The listing builds one solid part. Answer for the finished solid, in the listing's coordinates (mm). Round coordinates to 2 decimals unless told otherwise and drop trailing zeros. Order: outer loops, then holes, each group sorted by start corner. A loop starts at its lowest first (then second) coordinate and runs counter-clockwise, first axis right, second up. Notation, with made-up numbers: (44, -9) -> (82, -9) arc R10 ccw to (82, 7) -> close; hole circle Ø5 at (5.5, 12.5). An arc over 180 degrees is marked (long way). Answer in a Markdown table with one row per item. Add a question column.
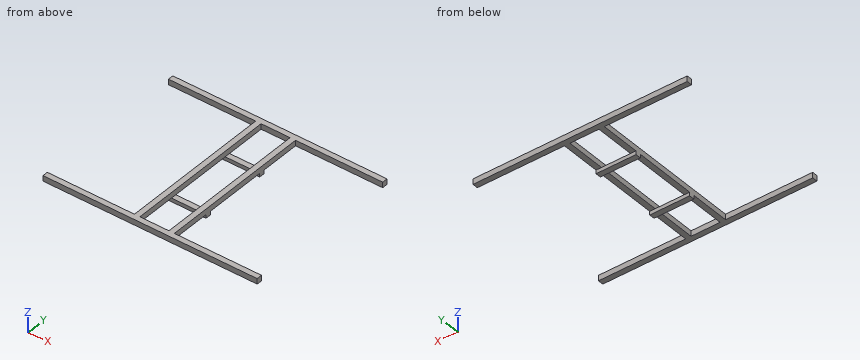
```python
from build123d import *

# Parameters (mm, degrees)
SKETCH1_W        = 110
SKETCH1_H        = 15
EXTRUDE1_DEPTH   = 10
EXTRUDE1_2_DEPTH = 10
SKETCH2_W        = 80
SKETCH2_H        = 421.99984649
EXTRUDE2_DEPTH   = 15


with BuildPart() as part:
    # Sketch1 → Extrude1 (new body)
    with BuildSketch(Plane.XY):
        with Locations((0, 93.499923245)):
            Rectangle(SKETCH1_W, SKETCH1_H)
    extrude(amount=EXTRUDE1_DEPTH)



with BuildPart() as body_2:
    # Sketch1 → Extrude1 2 (new body)
    with BuildSketch(Plane.XY):
        with Locations((0, -93.499923245)):
            Rectangle(SKETCH1_W, SKETCH1_H)
    extrude(amount=EXTRUDE1_2_DEPTH)


with BuildPart() as part_1:
    add(part.part)

    add(body_2.part)  # Extrude2 merges body 2
    # Sketch2 → Extrude2 (add)
    with BuildSketch(Plane.XY.offset(10)):
        Polygon((55, -210.999923245), (55, 210.999923245), (295, 210.999923245), (295, 225.999923245), (-295, 225.999923245), (-295, 210.999923245), (-55, 210.999923245), (-55, -210.999923245), (-295, -210.999923245), (-295, -225.999923245), (295, -225.999923245), (295, -210.999923245), align=None)
        Rectangle(SKETCH2_W, SKETCH2_H, mode=Mode.SUBTRACT)
    extrude(amount=EXTRUDE2_DEPTH)


solid = part_1.part
```
1. The part is cut by section B-B (z = 21). Give the vertices of the cut face in (x, y), then the cut area to 3 significant figures.
2. Each of these flat-tipped pins is pushed along its axis until it touches: pin 1 (7.5 mm diameter, centred on y = 84.5, z = 13, fed in from -X); pin 2 (3 mm diameter, centred on y = -168.5, z = 13, fed in from +X); pin 3 (5 mm diameter, centred on x = 23, z = 2.5, fed in from +Y). Where does it stop, or does it pass through?
3. Straight lines are drawn through the part: line 1 along Y through (x, z) = (-71.5, 21.5); line 2 along X through (y, z) = (-2.5, 21.75); line 3 along Z through (x, y) = (-22.5, 88). For each, find the intervals that lie inside material, in ascending order.
4. The part is cut by section C-C (x = 241.5). Give the vertices of the cut face in (y, z).
5. The part is cut by section A-A (x = -20.5). Give the vertices of the cut face in (y, z).
6. The part is cut by section D-D (y = -7.5). Give the vertices of the cut face in (x, z).
Report:
| question | item | result |
|---|---|---|
| 1 | outline | (-295, -226) -> (295, -226) -> (295, -211) -> (55, -211) -> (55, 211) -> (295, 211) -> (295, 226) -> (-295, 226) -> (-295, 211) -> (-55, 211) -> (-55, -211) -> (-295, -211) -> close; hole (-40, -211) -> (40, -211) -> (40, 211) -> (-40, 211) -> close |
| 1 | area | 30,400 mm^2 |
| 2 | pin 1 | stops at x = -55 |
| 2 | pin 2 | stops at x = 55 |
| 2 | pin 3 | stops at y = 101 |
| 3 | line 1 | y = -226 to -211, 211 to 226 |
| 3 | line 2 | x = -55 to -40, 40 to 55 |
| 3 | line 3 | z = 0 to 10 |
| 4 | outline | (-226, 10) -> (-211, 10) -> (-211, 25) -> (-226, 25) -> close; (211, 10) -> (226, 10) -> (226, 25) -> (211, 25) -> close |
| 5 | outline | (-226, 10) -> (-211, 10) -> (-211, 25) -> (-226, 25) -> close; (-101, 0) -> (-86, 0) -> (-86, 10) -> (-101, 10) -> close; (86, 0) -> (101, 0) -> (101, 10) -> (86, 10) -> close; (211, 10) -> (226, 10) -> (226, 25) -> (211, 25) -> close |
| 6 | outline | (-55, 10) -> (-40, 10) -> (-40, 25) -> (-55, 25) -> close; (40, 10) -> (55, 10) -> (55, 25) -> (40, 25) -> close |
